from build123d import *

# Parameters (mm, degrees)
F0_W      = 304.8
F0_H      = 355.6
F1_DEPTH  = 304.8
F2_W      = 254
F2_H      = 304.8
F3_DEPTH  = 304.801
F4_W      = 304.8
F4_H      = 254
F5_DEPTH  = 304.801
F6_W      = 254
F6_H      = 254
F7_DEPTH  = 25.4
F8_W      = 266.7
F8_H      = 266.7
F9_DEPTH  = 19.05
F10_W     = 279.4
F10_H     = 279.4
F11_DEPTH = 304.8
F12_R     = 4.7625
F13_DEPTH = 6.35
F16_DEPTH = 12.7
F19_DEPTH = 12.7
F20_R     = 8.526581
F21_DEPTH = 25.4


with BuildPart() as f1:
    # F0 (on Top) → F1 (new body)
    with BuildSketch(Plane.XY):
        with Locations((152.4, 177.8)):
            Rectangle(F0_W, F0_H)
    extrude(amount=F1_DEPTH)

    # F2 (on face) → F3 (cut, through all)
    with BuildSketch(Plane.XY.offset(304.8)):
        with Locations((152.4, 177.8)):
            Rectangle(F2_W, F2_H)
    extrude(amount=-F3_DEPTH, mode=Mode.SUBTRACT)

    # F4 (on face) → F5 (cut, through all)
    with BuildSketch(Plane.YZ.offset(304.8)):
        with Locations((177.8, 152.4)):
            Rectangle(F4_W, F4_H)
    extrude(amount=-F5_DEPTH, mode=Mode.SUBTRACT)

    # F6 (on face) → F7 (cut)
    with BuildSketch(Plane(origin=(0, 355.6, 0), x_dir=(-1, 0, 0), z_dir=(0, 1, 0))):
        with Locations((-152.4, 152.4)):
            Rectangle(F6_W, F6_H)
    extrude(amount=-F7_DEPTH, mode=Mode.SUBTRACT)

    # F8 (on face) → F9 (cut)
    with BuildSketch(Plane.XZ):
        with Locations((152.4, 152.4)):
            Rectangle(F8_W, F8_H)
    extrude(amount=-F9_DEPTH, mode=Mode.SUBTRACT)

    # F10 (on face) → F11 (cut)
    with BuildSketch(Plane(origin=(0, 25.4, 0), x_dir=(-1, 0, 0), z_dir=(0, 1, 0))):
        with Locations((-152.4, 152.4)):
            Rectangle(F10_W, F10_H)
    extrude(amount=F11_DEPTH, mode=Mode.SUBTRACT)

    # F12 (on face) → F13 (cut)
    with BuildSketch(Plane.XZ.offset(-19.05)):
        with Locations((31.75, 273.05)):
            Circle(F12_R)
        with Locations((273.05, 273.05)):
            Circle(F12_R)
        with Locations((273.05, 31.75)):
            Circle(F12_R)
        with Locations((31.75, 31.75)):
            Circle(F12_R)
    extrude(amount=-F13_DEPTH, mode=Mode.SUBTRACT)

    # F15 (on offset) → F16 (join, symmetric)
    with BuildSketch(Plane.YZ.offset(127)):
        Polygon((355.6, 25.4), (355.6, 0), (551.994091, 113.388181), (551.994091, 191.411819), (355.6, 304.8), (355.6, 279.4), (508, 191.411819), (508, 113.388181), align=None)
    extrude(amount=F16_DEPTH, both=True)

    # F18 (on offset) → F19 (join, symmetric)
    with BuildSketch(Plane.YZ.offset(177.8)):
        Polygon((355.6, 25.4), (355.6, 0), (551.470828, 113.086075), (551.470828, 191.713925), (355.6, 304.8), (355.6, 279.4), (507.476737, 191.713925), (507.476737, 113.086075), align=None)
    extrude(amount=F19_DEPTH, both=True)

    # F20 (on face) → F21 (join)
    with BuildSketch(Plane(origin=(165.1, 0, 0), x_dir=(0, -1, 0), z_dir=(-1, 0, 0))):
        with Locations((-528.486431, 152.795911)):
            Circle(F20_R)
    extrude(amount=F21_DEPTH)


solid = f1.part
Check sheet for the modelled part. Datum: model origin and axes. Units: mm. A direction names the side the tool comes from. Give positions to 0.01 mm unless a question says otherwise; leave off trailing zeros. Write each loop counter-clockwise with the first axis right and the second up, starting at its lowest first coordinate (ties: lowest second). Pieces come first, ordered by that corner, then holes. Notation, with made-up numbers: M 75,61.5 L 115,61.5 A17 ccw 115,90.5 Z; hole C 66,84 d8. An arc over 180 degrees is marked long. Use one line per item in the form item = value.
(1) Tool access check on faces 1 (the flat face through (12.7, 176, 19)), 2 (the flat face through (25.4, 176, 299)), 3 (the flat face through (151, 19.05, 154)), 4 (the flat face through (285, 355.6, 150)), 5 (the flat face through (177.978, 432.602, 69.857)). Record the directions out of +Z, -Z, +X, -X, +Y, -Y that give a thin tool (end or side, any length) a straight path to the whole face; none if there is none.
Answer block:
face_1 = none
face_2 = +Z, -Z
face_3 = -Y
face_4 = +Z, -Z, +X, +Y
face_5 = +X, -X
(2) Section check B-B on x = 252. Record the boundary of the cut face in (y, z), plus the area to 3 significant figures.
Answer block:
outline = M 0,0 L 25.4,0 L 25.4,304.8 L 0,304.8 L 0,285.75 L 19.05,285.75 L 19.05,19.05 L 0,19.05 Z; M 330.2,0 L 355.6,0 L 355.6,25.4 L 330.2,25.4 Z; M 330.2,279.4 L 355.6,279.4 L 355.6,304.8 L 330.2,304.8 Z
area = 3,950 mm2
(3) Section check A-A on y = 110. Record the boundary of the cut face in (x, z), plus the area to 3 significant figures.
Answer block:
outline = M 0,0 L 25.4,0 L 25.4,12.7 L 12.7,12.7 L 12.7,25.4 L 0,25.4 Z; M 0,279.4 L 12.7,279.4 L 12.7,292.1 L 25.4,292.1 L 25.4,304.8 L 0,304.8 Z; M 279.4,0 L 304.8,0 L 304.8,25.4 L 292.1,25.4 L 292.1,12.7 L 279.4,12.7 Z; M 279.4,292.1 L 292.1,292.1 L 292.1,279.4 L 304.8,279.4 L 304.8,304.8 L 279.4,304.8 Z
area = 1,940 mm2
(4) Section check D-D on y = 459.5. Record the boundary of the cut face in (x, z), plus the area to 3 significant figures.
Answer block:
outline = M 114.3,59.99 L 139.7,59.99 L 139.7,85.39 L 114.3,85.39 Z; M 114.3,219.41 L 139.7,219.41 L 139.7,244.81 L 114.3,244.81 Z; M 165.1,59.99 L 190.5,59.99 L 190.5,85.39 L 165.1,85.39 Z; M 165.1,219.41 L 190.5,219.41 L 190.5,244.81 L 165.1,244.81 Z
area = 2,580 mm2
(5) Section check C-C on z = 88. Record the boundary of the cut face in (x, y).
Answer block:
outline = M 0,0 L 19.05,0 L 19.05,19.05 L 285.75,19.05 L 285.75,0 L 304.8,0 L 304.8,25.4 L 0,25.4 Z; M 0,330.2 L 25.4,330.2 L 25.4,355.6 L 0,355.6 Z; M 114.3,464.03 L 139.7,464.03 L 139.7,508.02 L 114.3,508.02 Z; M 165.1,464.03 L 190.5,464.03 L 190.5,508.02 L 165.1,508.02 Z; M 279.4,330.2 L 304.8,330.2 L 304.8,355.6 L 279.4,355.6 Z
(6) Draft check along Z on faces 6 (the flat face through (178, 551.471, 152)), 7 (the flat face through (19, 176, 292.1)), 8 (the cylindrical face through (152.578, 535.253, 147.608)). Enter one of: pulls with the +Z half, pulls with the -Z half, needs draft (parallel to the pull), parting line crosses it, or undercut.
Answer block:
face_6 = needs draft
face_7 = undercut
face_8 = parting line crosses it
(7) Depth check by flat-ended pin: P1, Ø7.5, axis at x = 154.5, z = 10.5, coming from the +Y side; P2, Ø1, axis at x = 63, z = 192, coming from the -Y side; P3, Ø4, axis at x = 253.5, z = 105, coming from the +Y side. Enter the tip coordinate at first touch or a pass-through.
Answer block:
P1 = 355.6
P2 = 19.05
P3 = 25.4
(8) Material ranges on line 1 along X through (y, z) = (21, 273); line 2 along Z through (x, y) = (31, 21); line 3 along Y through (x, z) = (107.5, 283), recorded low to high.
Answer block:
line_1 = 0 to 26.99, 36.51 to 268.29, 277.81 to 304.8
line_2 = 0 to 27.05, 36.45 to 268.35, 277.75 to 304.8
line_3 = 19.05 to 25.4, 330.2 to 355.6
